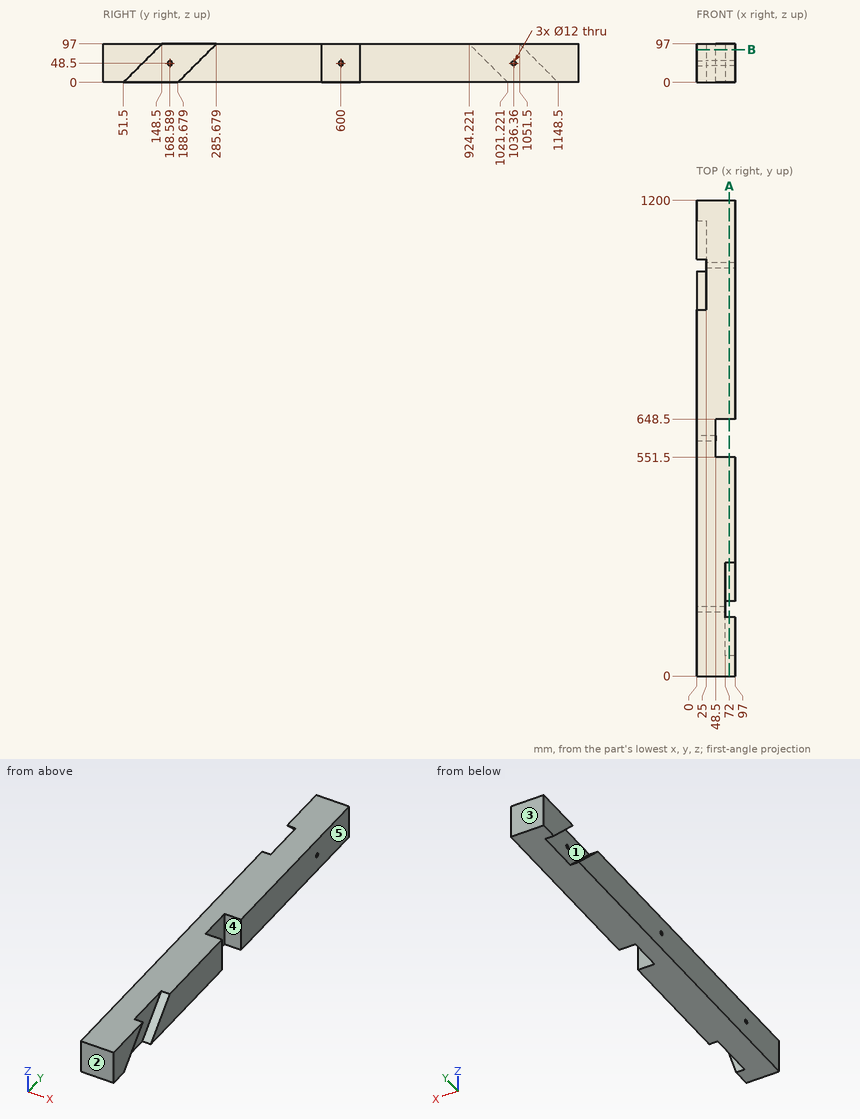
Check sheet for the drawn part. Datum: minimum x, y, z corner. Units: mm. A direction names the side the tool comes from. Round coordinates to 2 decimals unless told otherwise and drop trailing zeros. Order: outer loops, then holes, each group sorted by start corner. A loop starts at its lowest first (then second) coordinate and runs counter-clockwise, first axis right, second up. Notation, with made-up numbers: (47.25, 58) -> (76.25, 58) arc R11 ccw to (76.25, 71) -> close; hole circle Ø11 at (-33, 53). An arc over 180 degrees is marked (long way). Put each result on its own line as item: value. Start each with the question number.
(1) Material ranges on line 1 along Y through (x, z) = (71, 48); line 2 along Y through (x, z) = (26, 48); line 3 along Z through (x, y) = (10, 600), recorded low to high.
(2) Draft check along Y on the marked faces 3, 4 and 5. Enter one of: +Y half, -Y half, draft (parallel to the pull), parting line (faces both ways), or undercut.
(3) Tool access check on the marked faces 1 and 2. Record the directions out of +Z, -Z, +X, -X, +Y, -Y that give a thin tool (end or side, any length) a straight path to the whole face; none if there is none.
(4) Section check A-A (x = 83). Enter the section's corners in (y, z).
(5) Depth check by flat-ended pin: pin 1 Ø12 at (x, z) = (45, 81) entering from -Y; pin 2 Ø7 at (y, z) = (168.59, 48.5) entering from -X; pin 3 Ø15.5 at (y, z) = (600, 48.5) entering from +X; pin 4 Ø19 at (y, z) = (1036.36, 48.5) entering from -X. Enter the tip coordinate at first touch or a pass-through.
(6) Section check B-B (z = 83). Enter the section's corners in (x, y).
Completed:
1. line 1: y = 0 to 162.61, 174.57 to 551.5, 648.5 to 1030.38, 1042.34 to 1200
1. line 2: y = 0 to 162.61, 174.57 to 594.02, 605.98 to 1030.38, 1042.34 to 1200
1. line 3: z = 0 to 42.5, 54.5 to 97
2. face 3: +Y half
2. face 4: undercut
2. face 5: draft
3. face 1: -X
3. face 2: +Z, -Z, +X, -X, -Y
4. outline: (0, 0) -> (51.5, 0) -> (148.5, 97) -> (0, 97) -> close; (188.68, 0) -> (551.5, 0) -> (551.5, 97) -> (285.68, 97) -> close; (648.5, 0) -> (1200, 0) -> (1200, 97) -> (648.5, 97) -> close; hole circle Ø12 at (1036.36, 48.5)
5. pin 1: stops at y = 0
5. pin 2: passes through
5. pin 3: stops at x = 48.5
5. pin 4: stops at x = 25
6. outline: (0, 0) -> (97, 0) -> (97, 134.5) -> (72, 134.5) -> (72, 271.68) -> (97, 271.68) -> (97, 551.5) -> (48.5, 551.5) -> (48.5, 648.5) -> (97, 648.5) -> (97, 1200) -> (0, 1200) -> (0, 1065.5) -> (25, 1065.5) -> (25, 938.22) -> (0, 938.22) -> close
